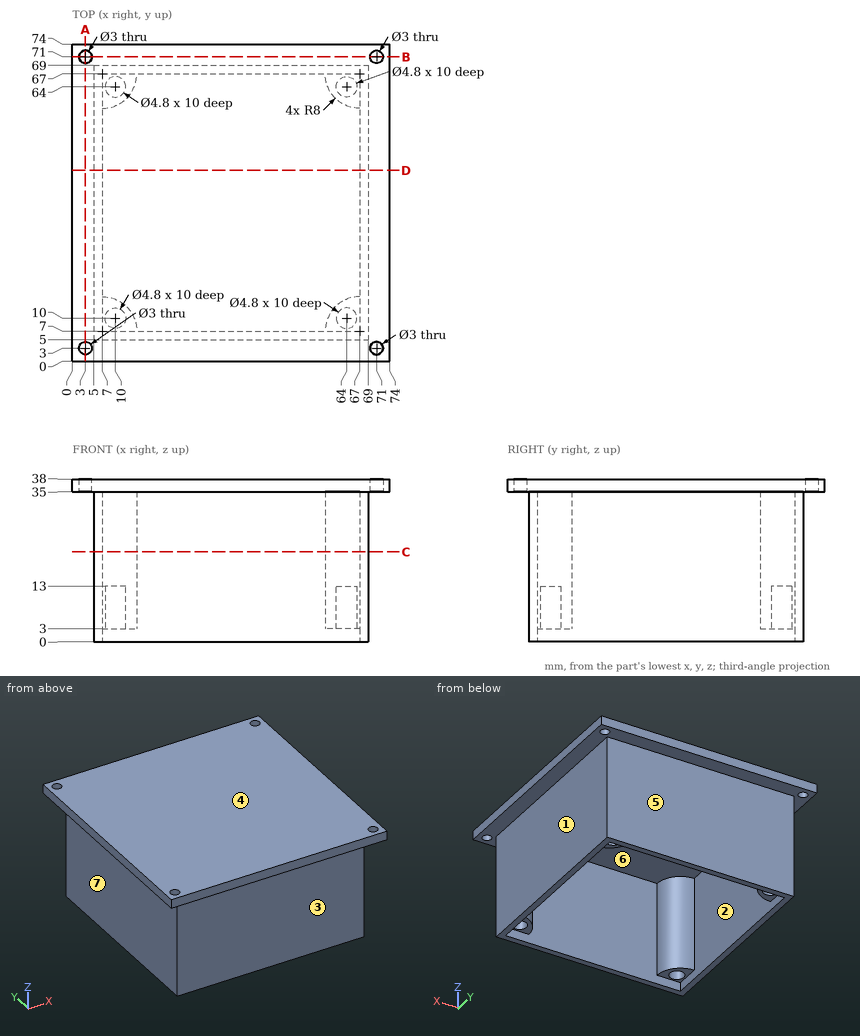
Geometry check sheet. Reference: drawing and pictorial views, mm from the part's lowest x, y, z. A direction names the side the tool comes from. Give positions to 0.01 mm unless a question says otherwise; leave off trailing zeros. Write each loop counter-clockwise with the first axis right and the second up, starting at its lowest first coordinate (ties: lowest second). Pieces come first, ordered by that corner, then holes. Notation, with made-up numbers: (-3.75, -17.5) - (6.25, -17.5) arc R31 ccw to (6.25, 16.5) - close; hole circle Ø6 at (71.25, -14.75). An arc over 180 degrees is marked (long way). Put each result on its own line as item: value.
Q1. Depth check by flat-ended pin: P1, Ø17.5, axis at x = 42.5, z = 24, coming from the +Y side; P2, Ø2.5, axis at x = 10, y = 64.5, coming from the -Z side; P3, Ø2, axis at x = 42.5, y = 61.5, coming from the -Z side; P4, Ø2.5, axis at x = 71, y = 71, coming from the -Z side (3 decimals). Enter the tip coordinate at first touch or a pass-through.
Result:
P1: y = 69
P2: z = 13
P3: z = 35
P4: through
Q2. Section check A-A on x = 3. Record the cut outline in (y, z).
Result:
outline: (0, 35) - (1.5, 35) - (1.5, 38) - (0, 38) - close; (4.5, 35) - (69.5, 35) - (69.5, 38) - (4.5, 38) - close; (72.5, 35) - (74, 35) - (74, 38) - (72.5, 38) - close
Q3. Scan lines: probe 1 along Y at (x, z) = (3, 37); probe 2 along Y at (x, z) = (35.5, 14). Record each from-to range of solid material in increasing order. Write a range as from..to.
Result:
probe 1: 0..1.5, 4.5..69.5, 72.5..74
probe 2: 5..7, 67..69
Q4. Section check C-C on z = 21. Record the cut outline in (x, y), and give its area (3 significant figures).
Result:
outline: (5, 5) - (69, 5) - (69, 69) - (5, 69) - close; hole (7, 15) arc R8 cw to (15, 7) - (59, 7) arc R8 cw to (67, 15) - (67, 59) arc R8 cw to (59, 67) - (15, 67) arc R8 cw to (7, 59) - close
area: 697 mm2
Q5. Set-up check for the marked faces 1, 2, 3 and 4: record each of +Z, -Z, +X, -X, +Y, -Y from which the full face is reachable in a straight line by a thin tool's end or side.
Result:
face 1: -Z, +X, +Y, -Y
face 2: -Z
face 3: -Z, +X, -X, -Y
face 4: +Z, +X, -X, +Y, -Y
Q6. Section check D-D on y = 44.5. Record the cut outline in (x, z).
Result:
outline: (0, 35) - (5, 35) - (5, 0) - (7, 0) - (7, 35) - (67, 35) - (67, 0) - (69, 0) - (69, 35) - (74, 35) - (74, 38) - (0, 38) - close
Q7. Mould release check, pull along X, two halves, no side actions. Record for the marked faces 5, 6 and 7: released by +X, released by -X, zero draft, split by the parting line, or undercut.
Result:
face 5: zero draft
face 6: undercut
face 7: released by -X
